Autodesk Inventor part; units mm, degrees
ref_plane "YZ Plane" through (0, 0, 0) normal (1, 0, 0) x (0, 1, 0)
ref_plane "XZ Plane" through (0, 0, 0) normal (0, 1, 0) x (-1, 0, 0)
ref_plane "XY Plane" through (0, 0, 0) normal (0, 0, 1) x (1, 0, 0)
sketch "Sketch1" plane through (0, 0, 0) normal (0, 1, 0) x (-1, 0, 0)
  line L0 (43, 0) -> (-43, 0) construction
  line L1 (43, 21) -> (-43, 21)
  line L2 (-43, -21) -> (43, -21)
  arc A0 (43, -21) -> (43, 21) centre (43, 0) ccw
  arc A1 (-43, 21) -> (-43, -21) centre (-43, 0) ccw
  point P0 (0, 0)
  dimension "d0" = 43
  dimension "d1" = 21
extrude "Extrusion1" add sketch "Sketch1" along normal blind 16
sketch "Sketch2" plane through (0, 16, 0) normal (0, 1, 0) x (1, 0, 0)
  arc A0 (43, -21) -> (43, 21) centre (43, 0) ccw
  arc A1 (-43, 21) -> (-43, -21) centre (-43, 0) ccw
  line L0 (-62.4165, 8) -> (-43, 8)
  arc A2 (-43, -8) -> (-43, 8) centre (-43, 0) ccw
  line L1 (-43, -8) -> (-62.4165, -8)
  line L2 (0, 29.4) -> (0, -29.4) construction
  line L3 (62.4165, 8) -> (43, 8)
  arc A3 (43, 8) -> (43, -8) centre (43, 0) ccw
  line L4 (43, -8) -> (62.4165, -8)
  point P0 (0, 0)
  dimension "d4" = 8
extrude "Extrusion2" cut sketch "Sketch2" against normal through all
sketch "Sketch3" plane through (0, 0, 0) normal (0, 1, 0) x (-1, 0, 0)
  line L0 (35, -39) -> (-35, -39)
  line L1 (-35, -39) -> (-35, -24)
  line L2 (-35, -24) -> (35, -24)
  line L3 (35, -24) -> (35, -39)
  line L4 (43, 21) -> (-43, 21)
  point P0 (0, 0)
  point P1 (0, -24)
  point P2 (0, 21)
  dimension "d7" = 70
  dimension "d8" = 15
  dimension "d9" = 60
extrude "Extrusion3" add sketch "Sketch3" along normal blind 62
sketch "Sketch4" plane through (0, 16, 0) normal (0, 1, 0) x (1, 0, 0)
  line L0 (43, 21) -> (-43, 21)
  line L1 (-35, 24) -> (35, 24)
  line L2 (-35, 24) -> (35, 24)
  line L3 (35, 24) -> (35, 21)
  line L4 (35, 21) -> (-35, 21)
  line L5 (-35, 21) -> (-35, 24)
  point P0 (0, 0)
extrude "Extrusion4" add sketch "Sketch4" against normal up to surface (16 mm away)
sketch "Sketch5" plane through (0, 62, 0) normal (0, 1, 0) x (1, 0, 0)
  line L0 (35, 39) -> (-35, 39)
  line L1 (-11, 34) -> (11, 34)
  line L2 (11, 34) -> (11, 22)
  line L3 (11, 22) -> (-11, 22)
  line L4 (-11, 22) -> (-11, 34)
  point P0 (0, 0)
  point P1 (0, 22)
  dimension "d14" = 5
  dimension "d15" = 22
  dimension "d16" = 12
extrude "Extrusion5" cut sketch "Sketch5" against normal through all
sketch "Sketch6" plane through (-43, 0, 21) normal (0, 0, 1) x (1, 0, 0)
  line L0 (0, 0) -> (86, 0)
  line L1 (0, 16) -> (86, 16)
  line L2 (32, 16) -> (54, 16)
  line L3 (54, 16) -> (54, 8)
  line L4 (54, 8) -> (32, 8)
  line L5 (32, 8) -> (32, 16)
  line L6 (32, 16) -> (32, 62)
  line L7 (54, 62) -> (54, 16)
  point P0 (43, 0)
  dimension "d19" = 8
extrude "Extrusion6" cut sketch "Sketch6" against normal up to surface (55 mm away)
sketch "Sketch7" plane through (-11, 62, -24) normal (1, 0, 0) x (0, 0, -1)
  line L0 (0, -46) -> (0, 0)
  line L1 (-45, -46) -> (0, -46)
  arc A0 (-5, -46) -> (0, -41) centre (-5, -41) ccw
  point P0 (-24, -62)
  dimension "d22" = 5
extrude "Extrusion7" add sketch "Sketch7" against normal up to surface (24 mm away)
mirror "Mirror1" about plane through (0, 0, 0) normal (1, 0, 0) of "Extrusion7"
fillet "Fillet1" radius 5 2 edges at (35, 8, -21) (-35, 8, -21)
sketch "Sketch8" plane through (-35, 62, -24) normal (0, 0, 1) x (1, 0, 0)
  line L0 (10, -24) -> (60, -24) construction
  line L1 (70, -62) -> (0, -62)
  point P0 (35, -62)
  point P1 (35, -24)
  dimension "d26" = 50
  dimension "d27" = 38
hole "Hole1" at (-25, 38, -24) at (25, 38, -24) direction (0, 0, -1) diameter 12 end through all
properties part number "Part022. Corner piece" material "Steel, Cast"
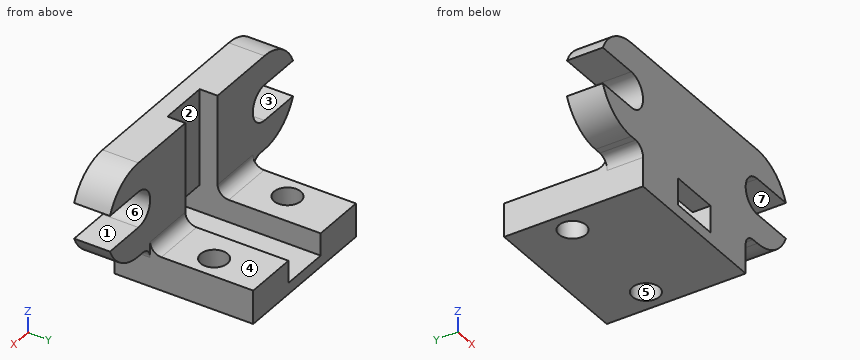
The model under review builds one solid part; all positions refer to its coordinate system, in mm. Face numbers are marked on the shaded views. A direction names the side the tool comes from. Round coordinates to 2 decimals unless told otherwise and drop trailing zeros. Write each loop counter-clockwise with the first axis right and the second up, starting at its lowest first coordinate (ties: lowest second). Pieces come first, ordered by that corner, then holes.
(1) We need section D-D on y = 37. Give the boundary of the cut face in (x, z).
(2) Mouldability with a two-part tool opening along X and no side actions: class the marked faces 5, 6 and 7 as +X half, -X half, draft (parallel to the pull), parting line (faces both ways), or undercut.
(3) We need section A-A on x = -5.5. Give the boundary of the cut face in (y, z).
(4) We need section B-B on z = 0. Give the boundary of the cut face in (x, y).
(5) Machinability: for the marked faces 1, 2, 3 and 4, which of the approach directions +Z, -Z, +X, -X, +Y, -Y give a long, thin tool a straight path to every point of the face, cutting with its end or side? Answer none if there is none.
(6) Insertion check: pin 1 (6 mm diameter, centred on x = 3.5, y = 18, fed in from +Z); pin 2 (8 mm diameter, centred on x = 55.5, y = 9.5, fed in from +Z); pin 3 (19 mm diameter, centred on x = -21.5, y = 41.5, fed in from +Z); pin 4 (6 mm diameter, centred on x = -44.5, z = -8.5, fed in from -Y). Each pin has a flat end and moves straight along its axis. Give the tip position at first contact, or say it passes through.
(7) Wall thickness on L1, parallel to X at y = 38, z = -33; L2, parallel to X at y = 38, z = -35.25; L3, parallel to X at y = 45.5, z = -25: over which ranges is each line inside the solid? List them lowest first.
(8) We need section C-C on x = 14. Give the boundary of the cut face in (y, z).
Findings below:
1. outline: (-35, -39) - (-30.92, -39) - (-30.92, -24) - (-35, -24) - close; (-19.08, -39) - (19.08, -39) - (19.08, -24) - (11, -24) - (11, -34) - (-11, -34) - (-11, -24) - (-19.08, -24) - close; (30.92, -39) - (35, -39) - (35, -24) - (30.92, -24) - close
2. face 5: undercut
2. face 6: +X half
2. face 7: draft
3. outline: (0, -39) - (62, -39) - (62, -34) - (0, -34) - close; (0, -22) - (8, -22) - (8, 21) - (0, 21) - close
4. outline: (-35, 0) - (35, 0) - (35, 16) - (11, 16) - (11, 8) - (-11, 8) - (-11, 16) - (-35, 16) - close
5. face 1: +X, +Y, -Y
5. face 2: +Z, +Y
5. face 3: -X, +Y, -Y
5. face 4: +Z, +X, -X, +Y
6. pin 1: stops at z = -34
6. pin 2: stops at z = 19.2
6. pin 3: stops at z = -24
6. pin 4: stops at y = 0
7. L1: x = -35 to -31, -19 to -11, 11 to 19, 31 to 35
7. L2: x = -35 to -31, -19 to 19, 31 to 35
7. L3: x = -35 to -11, 11 to 35
8. outline: (0, -39) - (62, -39) - (62, -24) - (21, -24) arc R5 cw to (16, -19) - (16, 21) - (0, 21) - close
